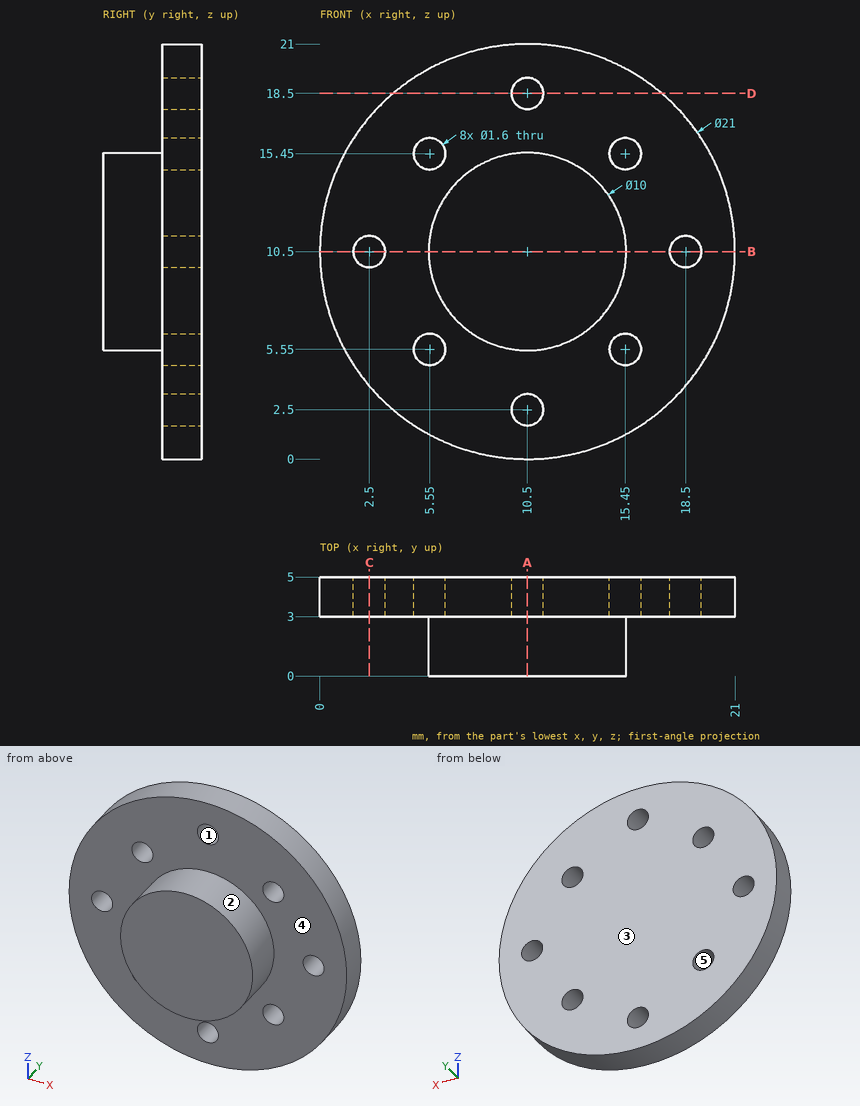
Here's the drawing with two shaded views (mm, measured from the low corner). I have some questions. A direction names the side the tool comes from. Give positions to 0.01 mm unless a question says otherwise; leave off trailing zeros. Order: outer loops, then holes, each group sorted by start corner. A loop starts at its lowest first (then second) coordinate and runs counter-clockwise, first axis right, second up. Notation, with made-up numbers: (-7, 39.25) - (24, 39.25) arc R11 ccw to (24, 55.25) - close; hole circle Ø4 at (57, -31). An arc over 180 degrees is marked (long way). Write each question's results on one line, items separated by ' | '.
1) I'm going to push flat-ended pins straight in: pin 1 Ø2 at (x, z) = (10.5, 2.5) entering from -Y; pin 2 Ø1.3 at (x, z) = (15.45, 15.45) entering from +Y. Where does each tip first touch, or does it pass through?
Final values:
pin 1: stops at y = 3 | pin 2: passes through
2) On a 3-axis mill with a long thin cutter (end or side, diameter ignored), from which of +Z, -Z, +X, -X, +Y, -Y can I reach the whole of each face in a straight line? I mean the marked faces 4 and 5. Say none if no direction works.
Final values:
face 4: -Y | face 5: +Y, -Y
3) Suppose I cut it at B-B, the plane z = 10.5. Write out the boundary of the cut face in (x, y), then the cut area to 3 significant figures.
Final values:
outline: (0, 3) - (1.7, 3) - (1.7, 5) - (0, 5) - close; (3.3, 3) - (5.5, 3) - (5.5, 0) - (15.5, 0) - (15.5, 3) - (17.7, 3) - (17.7, 5) - (3.3, 5) - close; (19.3, 3) - (21, 3) - (21, 5) - (19.3, 5) - close | area: 65.6 mm^2
4) Suppose I cut it at A-A, the plane x = 10.5. Write out the boundary of the cut face in (y, z), then the cut area to 3 significant figures.
Final values:
outline: (0, 5.5) - (3, 5.5) - (3, 3.3) - (5, 3.3) - (5, 17.7) - (3, 17.7) - (3, 15.5) - (0, 15.5) - close; (3, 0) - (5, 0) - (5, 1.7) - (3, 1.7) - close; (3, 19.3) - (5, 19.3) - (5, 21) - (3, 21) - close | area: 65.6 mm^2
5) If we mould it in two halves opening along X, with no side actions, what happens to the marked faces 1, 2 and 3? For each: pulls with the +X half, pulls with the -X half, needs draft (parallel to the pull), parting line crosses it, or undercut.
Final values:
face 1: undercut | face 2: parting line crosses it | face 3: needs draft
6) Please list where these lines run through material, in increasing order: line 1 along X through (y, z) = (4.4, 10.5); line 2 along Z through (x, y) = (5.5, 3.6); line 3 along Y through (x, z) = (3.75, 12). Write a range as [from, to].
Final values:
line 1: x = [0, 1.7], [3.3, 17.7], [19.3, 21] | line 2: z = [1.27, 4.75], [6.35, 14.65], [16.25, 19.73] | line 3: y = [3, 5]
7) Suppose I cut it at C-C, the plane x = 2.5. Write out the boundary of the cut face in (y, z), then the cut area to 3 significant figures.
Final values:
outline: (3, 3.7) - (5, 3.7) - (5, 9.7) - (3, 9.7) - close; (3, 11.3) - (5, 11.3) - (5, 17.3) - (3, 17.3) - close | area: 24.0 mm^2
8) Suppose I cut it at D-D, the plane z = 18.5. Write out the boundary of the cut face in (x, y).
Final values:
outline: (3.7, 3) - (9.7, 3) - (9.7, 5) - (3.7, 5) - close; (11.3, 3) - (17.3, 3) - (17.3, 5) - (11.3, 5) - close
